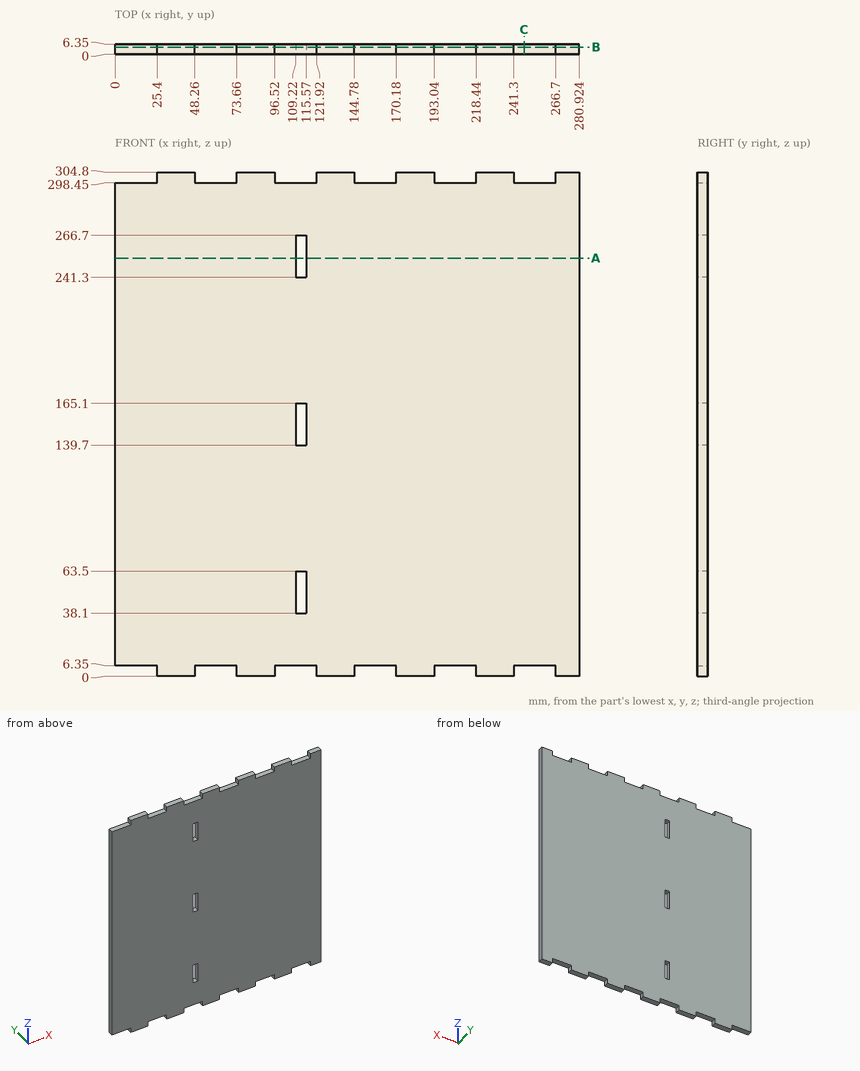
Check sheet for the drawn part. Datum: minimum x, y, z corner. Units: mm. Round coordinates to 2 decimals unless told otherwise and drop trailing zeros. Order: outer loops, then holes, each group sorted by start corner. A loop starts at its lowest first (then second) coordinate and runs counter-clockwise, first axis right, second up. Notation, with made-up numbers: M 3.25,38 L 54.25,38 A32 ccw 54.25,75 Z; hole C 41,50.5 d11. An arc over 180 degrees is marked long. Write each question's results on one line, items separated by ' | '. Start each with the question number.
1. Material ranges on L1, parallel to X at y = 1, z = 241.5; L2, parallel to Z at x = 256, y = 6.25, recorded low to high. Write a range as from..to.
2. Cross-section at A-A on z = 253. Record the boundary of the cut face in (x, y).
3. Cross-section at B-B on y = 4.5. Give the number of separate pieces and of enclosed holes in the cut face, plus the area to 3 significant figures.
4. Cross-section at C-C on x = 247.5. Record the boundary of the cut face in (y, z).
5. Go/stop test with flat-tipped pins: P1, Ø3, axis at x = 14.5, y = 2.5, coming from the -Z side; P2, Ø3, axis at y = 1.5, z = 4.5, coming from the -X side; P3, Ø1.5, axis at x = 163.5, y = 3.5, coming from the +Z side. Record where each tip stops, or that it passes through.
Resolved:
1) L1: 0..109.22, 115.57..280.92 | L2: 6.35..298.45
2) outline: M 0,0 L 109.22,0 L 109.22,6.35 L 0,6.35 Z; M 115.57,0 L 280.92,0 L 280.92,6.35 L 115.57,6.35 Z
3) separate pieces: 1 | enclosed holes: 3 | area: 83,200 mm2
4) outline: M 0,6.35 L 6.35,6.35 L 6.35,298.45 L 0,298.45 Z
5) P1: z = 6.35 | P2: x = 25.4 | P3: z = 298.45
